Source: CAD feature listing. Evaluate the final solid. Frame: model axes, mm. Give positions to 0.01 mm unless a question says otherwise; leave off trailing zeros. Write each loop counter-clockwise with the first axis right and the second up, starting at its lowest first coordinate (ties: lowest second). Pieces come first, ordered by that corner, then holes. Notation, with made-up numbers: (4, 35) -> (36, 35) arc R22 ccw to (36, 74) -> close; hole circle Ø10 at (13.5, 47.25). An arc over 180 degrees is marked (long way). Use a Markdown table: item, result. Add a question column.
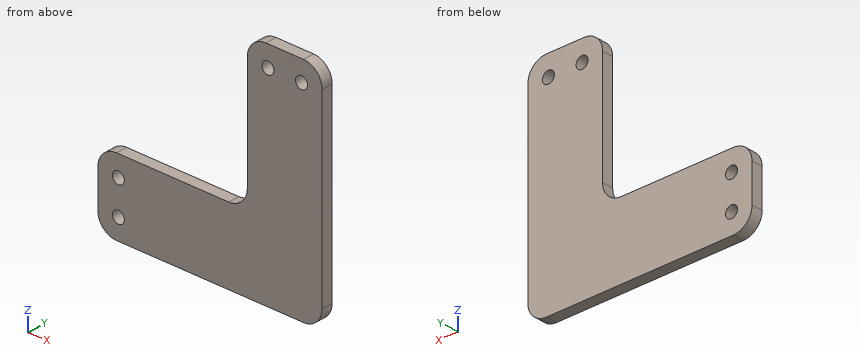
```python
from build123d import *

# Parameters (mm, degrees)
EXTRUDE_1_DEPTH     = 3
SKETCH_2_R          = 1.6
CUT_EXTRUDE_1_DEPTH = 65.101482042
FILLET_1_R          = 5


with BuildPart() as part:
    # 草图1 → 凸台-拉伸1 (new body)
    with BuildSketch(Plane(origin=(0, 0, 0), x_dir=(1, 0, 0), z_dir=(0, 1, 0))):
        Polygon((-50, 40), (-50, 20), (-10, 20), (-10, -20), (10, -20), (10, 40), align=None)
    extrude(amount=EXTRUDE_1_DEPTH)

    # 草图2 → 切除-拉伸1 (cut, through all)
    with BuildSketch(Plane(origin=(0, 3, 0), x_dir=(1, 0, 0), z_dir=(0, 1, 0))):
        with Locations(Location((-44.5, 34.5, 0), (0, 0, 270))):
            Circle(SKETCH_2_R)
        with Locations(Location((-44.5, 25.5, 0), (0, 0, 270))):
            Circle(SKETCH_2_R)
        with Locations(Location((-4.5, -14.5, 0), (0, 0, 270))):
            Circle(SKETCH_2_R)
        with Locations(Location((4.5, -14.5, 0), (0, 0, 270))):
            Circle(SKETCH_2_R)
    extrude(amount=-CUT_EXTRUDE_1_DEPTH, mode=Mode.SUBTRACT)

    # 圆角1
    fillet_1_edges = [part.edges().sort_by_distance(p)[0] for p in [
        (10, 1.5, 20),
        (-10, 1.5, 20),
        (-10, 1.5, -20),
        (-50, 1.5, -20),
        (-50, 1.5, -40),
        (10, 1.5, -40),
    ]]
    fillet(fillet_1_edges, radius=FILLET_1_R)


solid = part.part
```
(1) Cut plane B-B on z = -1. Return the cut outline in (x, y).
(2) Material intervals for L1, parallel to X at y = 0.8, z = 14.5; L2, parallel to X at y = 0.2, z = 15; L3, parallel to X at y = 0.6, z = -2.5, sorted ascending.
(3) First-contact query: pin 1 Ø3 at (x, z) = (4.5, 14.5) entering from +Y; pin 2 Ø0.9 at (x, y) = (-36.5, 1.5) entering from +Z; pin 3 Ø1 at (y, z) = (2.5, -14) entering from -X. Flat tips, straight axial feed; report the tip coordinate or a pass-through.
(4) Cut plane C-C on x = -28.5. Return the cut outline in (y, z).
(5) Cut plane A-A on y = 1.5. Return the cut outline in (x, z).
Output:
| question | item | result |
|---|---|---|
| 1 | outline | (-10, 0) -> (10, 0) -> (10, 3) -> (-10, 3) -> close |
| 2 | L1 | -10 to -6.1, -2.9 to 2.9, 6.1 to 10 |
| 2 | L2 | -10 to -6.02, -2.98 to 2.98, 6.02 to 10 |
| 2 | L3 | -10 to 10 |
| 3 | pin 1 | through |
| 3 | pin 2 | z = -20 |
| 3 | pin 3 | x = -10 |
| 4 | outline | (0, -40) -> (3, -40) -> (3, -20) -> (0, -20) -> close |
| 5 | outline | (-50, -35) arc R5 ccw to (-45, -40) -> (5, -40) arc R5 ccw to (10, -35) -> (10, 15) arc R5 ccw to (5, 20) -> (-5, 20) arc R5 ccw to (-10, 15) -> (-10, -15) arc R5 cw to (-15, -20) -> (-45, -20) arc R5 ccw to (-50, -25) -> close; hole circle Ø3.2 at (-44.5, -34.5); hole circle Ø3.2 at (-44.5, -25.5); hole circle Ø3.2 at (-4.5, 14.5); hole circle Ø3.2 at (4.5, 14.5) |
